```python
from build123d import *

# Parameters (mm, degrees)
F1_DEPTH = 1000
F2_R     = 10


with BuildPart() as f1:
    # F0 (on Right) → F1 (new body)
    with BuildSketch(Plane.YZ):
        with BuildLine():
            Line((-55, -12.5), (55, -12.5))
            Line((55, -12.5), (55, 2.5))
            ThreePointArc((55, 2.5), (52.0710678119, 9.5710678119), (45, 12.5))
            Line((45, 12.5), (-45, 12.5))
            ThreePointArc((-45, 12.5), (-52.0710678119, 9.5710678119), (-55, 2.5))
            Line((-55, 2.5), (-55, -12.5))
        make_face()
    extrude(amount=F1_DEPTH)

    # F2
    f2_edges = [f1.edges().sort_by_distance(p)[0] for p in [
        (1000, 0, 12.5),
        (500, 45, 12.5),
        (500, -45, 12.5),
        (0, 0, 12.5),
    ]]
    fillet(f2_edges, radius=F2_R)


solid = f1.part
```
Build history of the part. All positions in model axes, mm. Round coordinates to 2 decimals unless told otherwise and drop trailing zeros. Loops run counter-clockwise (first coordinate to the right, second up) from the corner with the lowest first, then second, coordinate; pieces in that order, holes last.
Item 1: Pin check, flat tips, straight feed: P1, Ø2, axis at x = 162.5, z = 8, coming from the -Y side; P2, Ø4, axis at x = 858.5, z = 9, coming from the +Y side. Stop position of each tip, or through.
Item 2: Saw through at A-A (x = 596). List the corners of the cut face in (y, z).
Item 3: Drill centre lines: line 1 along Z through (x, y) = (361.5, -46); line 2 along Y through (x, z) = (698, 3); line 3 along X through (y, z) = (-17, 11.75). Where is each one in solid material? Low to high.
Worked answers:
1. P1: stops at y = -53.93
1. P2: stops at y = 53.93
2. outline: (-55, -12.5) - (55, -12.5) - (55, 2.5) arc R10 ccw to (45, 12.5) - (-45, 12.5) arc R10 ccw to (-55, 2.5) - close
3. line 1: z = -12.5 to 12.45
3. line 2: y = -54.99 to 54.99
3. line 3: x = 6.2 to 993.8
